```python
from build123d import *

# Parameters (mm, degrees)
SKETCH_1_R          = 26
EXTRUDE_1_DEPTH     = 40
SKETCH_2_R          = 3.5
CUT_EXTRUDE_1_DEPTH = 67.5
SKETCH_3_W          = 33.659947674
SKETCH_3_H          = 4
CUT_EXTRUDE_3_DEPTH = 41
FILLET_1_R          = 1


with BuildPart() as part:
    # 草图1 → 凸台-拉伸1 (new body)
    with BuildSketch(Plane.XY):
        Polygon((-12.5, -33.25), (12.5, -33.25), (27.5, -19.35), (42.5, -19.35), (42.5, 13.25), (45, 15.75), (45, 33.25), (22.5, 33.25), (20.5, 31.25), (9.5, 31.25), (7.5, 33.25), (-7.5, 33.25), (-9.5, 31.25), (-20.5, 31.25), (-22.5, 33.25), (-45, 33.25), (-45, 15.75), (-42.5, 13.25), (-42.5, -19.35), (-27.5, -19.35), align=None)
        Circle(SKETCH_1_R, mode=Mode.SUBTRACT)
    extrude(amount=EXTRUDE_1_DEPTH)

    # 草图2 → 切除-拉伸1 (cut, through all)
    with BuildSketch(Plane(origin=(0, 33.25, 0), x_dir=(1, 0, 0), z_dir=(0, 1, 0))):
        with Locations((-35, -10)):
            Circle(SKETCH_2_R)
        with Locations((-35, -30)):
            Circle(SKETCH_2_R)
        with Locations((35, -30)):
            Circle(SKETCH_2_R)
        with Locations((35, -10)):
            Circle(SKETCH_2_R)
    extrude(amount=-CUT_EXTRUDE_1_DEPTH, mode=Mode.SUBTRACT)

    # 草图3 → 切除-拉伸3 (cut, through all)
    with BuildSketch(Plane.XY):
        with Locations((-31.784741675, 0)):
            Rectangle(SKETCH_3_W, SKETCH_3_H)
    extrude(amount=CUT_EXTRUDE_3_DEPTH, mode=Mode.SUBTRACT)

    # 圆角1
    fillet_1_edges = [part.edges().sort_by_distance(p)[0] for p in [
        (42.5, -19.35, 20),
        (-42.5, -19.35, 20),
    ]]
    fillet(fillet_1_edges, radius=FILLET_1_R)


solid = part.part
```
Verification items for the finished model (mm, model axes). A direction names the side the tool comes from. Coordinates: 2 decimals unless noted, no trailing zeros. Write each loop counter-clockwise with the first axis right and the second up, starting at its lowest first coordinate (ties: lowest second). Pieces come first, ordered by that corner, then holes. Notation, with made-up numbers: M -1.5,-3.75 L 47.5,-3.75 A12 cw 47.5,1.25 Z; hole C 28,15.5 d1. An arc over 180 degrees is marked long. One line per item, written item: value.
Item 1: Scan lines: line 1 along Z through (x, y) = (-35, -14.5); line 2 along Y through (x, z) = (-36, 5.5); line 3 along X through (y, z) = (7, 11.5). Record each from-to range of solid material in increasing order.
Check sheet entries:
line 1: z = 0 to 6.5, 13.5 to 26.5, 33.5 to 40
line 2: y = -19.35 to -2, 2 to 33.25
line 3: x = -42.5 to -38.16, -31.84 to -25.04, 25.04 to 31.84, 38.16 to 42.5
Item 2: Section check A-A, the plane x = -35. Record the boundary of the cut face in (y, z), plus the area to 3 significant figures.
Check sheet entries:
outline: M -19.35,0 L -2,0 L -2,6.5 L -19.35,6.5 Z; M -19.35,13.5 L -2,13.5 L -2,26.5 L -19.35,26.5 Z; M -19.35,33.5 L -2,33.5 L -2,40 L -19.35,40 Z; M 2,0 L 33.25,0 L 33.25,6.5 L 2,6.5 Z; M 2,13.5 L 33.25,13.5 L 33.25,26.5 L 2,26.5 Z; M 2,33.5 L 33.25,33.5 L 33.25,40 L 2,40 Z
area: 1,260 mm^2
Item 3: Access from +Z, -Z, +X, -X, +Y, -Y to the whole of each face (thin tool, end or side, straight path). Record for faces 1 (the flat face through (-42.5, 8, 20)), 2 (the flat face through (8.51, 32.24, 19.72)), 3 (the flat face through (34, -19.35, 20)).
Check sheet entries:
face 1: +Z, -Z, -X, -Y
face 2: +Z, -Z, +Y
face 3: +Z, -Z, +X, -Y
Item 4: Mould release check, pull along Z, two halves, no side actions. Record for faces 4 (the cylindrical face through (-35.46, -10.55, 26.53)), 5 (the flat face through (19.895, -26.397, 19.72)), 6 (the flat face through (-1, 30, 40)): pulls with the +Z half, pulls with the -Z half, needs draft (parallel to the pull), parting line crosses it, or undercut.
Check sheet entries:
face 4: undercut
face 5: needs draft
face 6: pulls with the +Z half
Item 5: Section check D-D, the plane y = -21. Record the boundary of the cut face in (x, z).
Check sheet entries:
outline: M -25.72,0 L -15.33,0 L -15.33,40 L -25.72,40 Z; M 15.33,0 L 25.72,0 L 25.72,40 L 15.33,40 Z
Item 6: Section check C-C, the plane x = 0. Record the boundary of the cut face in (y, z), plus the area to 3 significant figures.
Check sheet entries:
outline: M -33.25,0 L -26,0 L -26,40 L -33.25,40 Z; M 26,0 L 33.25,0 L 33.25,40 L 26,40 Z
area: 580 mm^2
Item 7: Gauge pin test, flat ends, axial feed: pin 1 Ø3.5 at (y, z) = (8, 14) entering from -X; pin 2 Ø8 at (y, z) = (-3.5, 9) entering from +X; pin 3 Ø10 at (x, z) = (18.5, 35) entering from -Y; pin 4 Ø5.5 at (x, z) = (35, 10) entering from -Y. Record the tip position at first contact, or that the pin passes through.
Check sheet entries:
pin 1: stops at x = -42.5
pin 2: stops at x = 42.5
pin 3: stops at y = -32.32
pin 4: passes through
Item 8: Section check B-B, the plane y = 23. Record the boundary of the cut face in (x, z).
Check sheet entries:
outline: M -45,0 L -12.12,0 L -12.12,40 L -45,40 Z; M 12.12,0 L 45,0 L 45,40 L 12.12,40 Z; hole C -35,10 d7; hole C -35,30 d7; hole C 35,10 d7; hole C 35,30 d7
